from build123d import *

# Parameters (mm, degrees)
SKETCH1_W           = 33
SKETCH1_H           = 17
BOSS_EXTRUDE1_DEPTH = 3
CUT_EXTRUDE1_DEPTH  = 4


with BuildPart() as part:
    # Sketch1 → Boss-Extrude1 (new body)
    with BuildSketch(Plane(origin=(0, 0, 0), x_dir=(1, 0, 0), z_dir=(0, 1, 0))):
        with Locations((16.5, 8.5)):
            Rectangle(SKETCH1_W, SKETCH1_H)
    extrude(amount=BOSS_EXTRUDE1_DEPTH)

    # Sketch2 → Cut-Extrude1 (cut, through all)
    with BuildSketch(Plane(origin=(0, 3, 0), x_dir=(1, 0, 0), z_dir=(0, 1, 0))):
        with BuildLine():
            Line((21.7, 11.3), (27.2, 11.3))
            ThreePointArc((27.2, 11.3), (30, 8.5), (27.2, 5.7))
            Line((27.2, 5.7), (21.7, 5.7))
            ThreePointArc((21.7, 5.7), (18.9, 8.5), (21.7, 11.3))
        make_face()
        with BuildLine():
            Line((6.95, 12), (6.95, 13.5))
            ThreePointArc((6.95, 13.5), (8.6, 15.15), (10.25, 13.5))
            Line((10.25, 13.5), (10.25, 12))
            ThreePointArc((10.25, 12), (8.6, 10.35), (6.95, 12))
        make_face()
        with BuildLine():
            Line((3.6, 10.15), (5.1, 10.15))
            ThreePointArc((5.1, 10.15), (6.75, 8.5), (5.1, 6.85))
            Line((5.1, 6.85), (3.6, 6.85))
            ThreePointArc((3.6, 6.85), (1.95, 8.5), (3.6, 10.15))
        make_face()
        with BuildLine():
            Line((13.6, 10.15), (12.1, 10.15))
            ThreePointArc((12.1, 10.15), (10.45, 8.5), (12.1, 6.85))
            Line((12.1, 6.85), (13.6, 6.85))
            ThreePointArc((13.6, 6.85), (15.25, 8.5), (13.6, 10.15))
        make_face()
        with BuildLine():
            Line((6.95, 5), (6.95, 3.5))
            ThreePointArc((6.95, 3.5), (8.6, 1.85), (10.25, 3.5))
            Line((10.25, 3.5), (10.25, 5))
            ThreePointArc((10.25, 5), (8.6, 6.65), (6.95, 5))
        make_face()
    extrude(amount=-CUT_EXTRUDE1_DEPTH, mode=Mode.SUBTRACT)


solid = part.part
Input: part model. Units: mm. Frame: model coordinates. A direction names the side the tool comes from. Give positions to 0.01 mm unless a question says otherwise; leave off trailing zeros. Loops run counter-clockwise (first coordinate to the right, second up) from the corner with the lowest first, then second, coordinate; pieces in that order, holes last. Notation, with made-up numbers: (-29, -8) - (5, -8) arc R8 ccw to (5, -2) - close; hole circle Ø1 at (17, -9). An arc over 180 degrees is marked (long way). Use CSV: the item, a comma, the result in double quotes. Start each with the question number.
Item 1: Section B-B on x = 4.5. Return loops of the section in (y, z).
Item 2: Section D-D on z = -9.5. Return loops of the section in (x, y), then the cut area to 3 significant figures.
Item 3: Reachability of faces 4 (the flat face through (16, 1, -17)), 5 (the flat face through (13, 2, -6.85)) from +Z, -Z, +X, -X, +Y, -Y: full face, straight path, thin tool, end or side. Return the list, or none.
Item 4: Mould query, pull axis Z, two halves, no side actions, for faces 1 (the cylindrical face through (10.45, 1.52, -8.54)), 2 (the flat face through (33, 1, -8)), 3 (the flat face through (16, 1, 0)). Classes: pulls with the +Z half, pulls with the -Z half, needs draft (parallel to the pull), parting line crosses it, or undercut.
Item 5: Line query: line 1 (Z direction, x = 22, y = 2.2); line 2 (Z direction, x = 5, y = 2.35); line 3 (Z direction, x = 8, y = 0.35). Output: solid intervals per line, ascending.
Item 6: Contact query for a flat-ended pin moving along its axis: P1, Ø2, axis at x = 8, z = -12, coming from the +Y side. Output: stop coordinate, or through.
Item 7: Section A-A on x = 8.6. Return loops of the section in (y, z), then the cut area to 3 significant figures.
Item 8: Section C-C on y = 2.25. Return loops of the section in (x, z).
Ans:
1,outline,"(0, -17) - (3, -17) - (3, -10.15) - (0, -10.15) - close; (0, -6.85) - (3, -6.85) - (3, 0) - (0, 0) - close"
2,outline,"(0, 0) - (2.29, 0) - (2.29, 3) - (0, 3) - close; (6.41, 0) - (10.79, 0) - (10.79, 3) - (6.41, 3) - close; (14.91, 0) - (19.08, 0) - (19.08, 3) - (14.91, 3) - close; (29.82, 0) - (33, 0) - (33, 3) - (29.82, 3) - close"
2,area,"42.1 mm2"
3,face 4,"-Z, +X, -X, +Y, -Y"
3,face 5,"+Y, -Y"
4,face 1,"undercut"
4,face 2,"needs draft"
4,face 3,"pulls with the +Z half"
5,line 1,"z = -17 to -11.3, -5.7 to 0"
5,line 2,"z = -17 to -10.15, -6.85 to 0"
5,line 3,"z = -17 to -15.04, -10.46 to -6.54, -1.96 to 0"
6,P1,"passes through"
7,outline,"(0, -17) - (3, -17) - (3, -15.15) - (0, -15.15) - close; (0, -10.35) - (3, -10.35) - (3, -6.65) - (0, -6.65) - close; (0, -1.85) - (3, -1.85) - (3, 0) - (0, 0) - close"
7,area,"22.2 mm2"
8,outline,"(0, -17) - (33, -17) - (33, 0) - (0, 0) - close; hole (3.6, -10.15) - (5.1, -10.15) arc R1.65 ccw to (5.1, -6.85) - (3.6, -6.85) arc R1.65 ccw to start; hole (6.95, -13.5) arc R1.65 ccw to (10.25, -13.5) - (10.25, -12) arc R1.65 ccw to (6.95, -12) - close; hole (6.95, -5) arc R1.65 ccw to (10.25, -5) - (10.25, -3.5) arc R1.65 ccw to (6.95, -3.5) - close; hole (12.1, -10.15) - (13.6, -10.15) arc R1.65 ccw to (13.6, -6.85) - (12.1, -6.85) arc R1.65 ccw to start; hole (21.7, -11.3) - (27.2, -11.3) arc R2.8 ccw to (27.2, -5.7) - (21.7, -5.7) arc R2.8 ccw to start"
